from build123d import *

# Parameters (mm, degrees)
F1_DEPTH = 254
F2_R     = 2
F3_R     = 5


with BuildPart() as f1:
    # F0 (on Right) → F1 (new body)
    with BuildSketch(Plane.YZ):
        Polygon((-11.62, 7.9759603159), (-15.94, 12.2959603159), (-15.94, -0.5893383893), (-11.62, -0.5893383893), align=None)
        Polygon((-11.62, 11.0306616107), (-15.94, 15.3506616107), (-15.94, 12.2959603159), (-11.62, 7.9759603159), (-8.7938307864, 5.1497911023), (-7.266480139, 6.6771417497), align=None)
        Polygon((-8.5652987053, 11.0306616107), (-11.62, 11.0306616107), (-7.266480139, 6.6771417497), (-5.7391294917, 8.2044923971), align=None)
        Polygon((0, 15.3506616107), (-12.8852987053, 15.3506616107), (-8.5652987053, 11.0306616107), (0, 11.0306616107), align=None)
        Polygon((-12.8852987053, 15.3506616107), (-15.94, 15.3506616107), (-11.62, 11.0306616107), (-8.5652987053, 11.0306616107), align=None)
        Polygon((-15.94, -21.5946370946), (-11.62, -17.2746370946), (-11.62, -8.7093383893), (-15.94, -8.7093383893), align=None)
        Polygon((-3.625, -12.3343383893), (-3.625, -9.2796370946), (-11.62, -17.2746370946), (-15.94, -21.5946370946), (-15.94, -24.6493383893), (-12.8852987053, -24.6493383893), (-8.5652987053, -20.3293383893), (-0.5702987053, -12.3343383893), align=None)
        Polygon((0, -20.3293383893), (-8.5652987053, -20.3293383893), (-12.8852987053, -24.6493383893), (0, -24.6493383893), align=None)
        Polygon((14.9650698751, 9.3104327805), (8.6902987053, 3.0356616107), (11.745, 3.0356616107), (11.745, -0.0190396841), (18.0197711699, 6.2557314858), (19.74, 7.9759603159), (16.6852987053, 11.0306616107), align=None)
        Polygon((21.0052987053, 15.3506616107), (16.6852987053, 11.0306616107), (19.74, 7.9759603159), (24.06, 12.2959603159), (24.06, 15.3506616107), align=None)
        Polygon((24.06, 12.2959603159), (19.74, 7.9759603159), (19.74, -0.5893383893), (24.06, -0.5893383893), align=None)
        Polygon((8.12, 11.0306616107), (16.6852987053, 11.0306616107), (21.0052987053, 15.3506616107), (8.12, 15.3506616107), align=None)
        with BuildLine():
            Line((11.745, -9.2796370946), (11.745, -0.0190396841))
            Line((11.745, -0.0190396841), (7.4440143218, -4.3200253623))
            ThreePointArc((7.4440143218, -4.3200253623), (7.456001229, -4.4844879937), (7.46, -4.6493383893))
            ThreePointArc((7.46, -4.6493383893), (7.456001229, -4.8141887849), (7.4440143218, -4.9786514164))
            Line((7.4440143218, -4.9786514164), (11.745, -9.2796370946))
        make_face()
        with BuildLine():
            Line((3.7306869729, -8.0333527111), (-0.5702987053, -12.3343383893))
            Line((-0.5702987053, -12.3343383893), (8.6902987053, -12.3343383893))
            Line((8.6902987053, -12.3343383893), (4.3893130271, -8.0333527111))
            ThreePointArc((4.3893130271, -8.0333527111), (4.06, -8.0493383893), (3.7306869729, -8.0333527111))
        make_face()
        with BuildLine():
            Line((0.6759856782, -4.3200253623), (-3.625, -0.0190396841))
            Line((-3.625, -0.0190396841), (-3.625, -9.2796370946))
            Line((-3.625, -9.2796370946), (0.6759856782, -4.9786514164))
            ThreePointArc((0.6759856782, -4.9786514164), (0.66, -4.6493383893), (0.6759856782, -4.3200253623))
        make_face()
        with BuildLine():
            Line((8.6902987053, 3.0356616107), (-0.5702987053, 3.0356616107))
            Line((-0.5702987053, 3.0356616107), (3.7306869729, -1.2653240675))
            ThreePointArc((3.7306869729, -1.2653240675), (4.06, -1.2493383893), (4.3893130271, -1.2653240675))
            Line((4.3893130271, -1.2653240675), (8.6902987053, 3.0356616107))
        make_face()
        Polygon((-5.7391294917, 8.2044923971), (-7.266480139, 6.6771417497), (-3.625, 3.0356616107), (-0.5702987053, 3.0356616107), align=None)
        Polygon((-3.625, 3.0356616107), (-7.266480139, 6.6771417497), (-8.7938307864, 5.1497911023), (-3.625, -0.0190396841), align=None)
        Polygon((11.745, -12.3343383893), (8.6902987053, -12.3343383893), (16.6852987053, -20.3293383893), (21.0052987053, -24.6493383893), (24.06, -24.6493383893), align=None)
        Polygon((19.74, -17.2746370946), (11.745, -9.2796370946), (11.745, -12.3343383893), (24.06, -24.6493383893), (24.06, -21.5946370946), align=None)
        Polygon((19.74, -8.7093383893), (19.74, -17.2746370946), (24.06, -21.5946370946), (24.06, -8.7093383893), align=None)
        Polygon((21.0052987053, -24.6493383893), (16.6852987053, -20.3293383893), (8.12, -20.3293383893), (8.12, -24.6493383893), align=None)
        with BuildLine():
            Line((11.745, 3.0356616107), (8.6902987053, 3.0356616107))
            Line((8.6902987053, 3.0356616107), (4.3893130271, -1.2653240675))
            ThreePointArc((4.3893130271, -1.2653240675), (6.464163056, -2.2451753333), (7.4440143218, -4.3200253623))
            Line((7.4440143218, -4.3200253623), (11.745, -0.0190396841))
            Line((11.745, -0.0190396841), (11.745, 3.0356616107))
        make_face()
        with BuildLine():
            Line((1.655836944, -2.2451753333), (-3.625, 3.0356616107))
            Line((-3.625, 3.0356616107), (-3.625, -0.0190396841))
            Line((-3.625, -0.0190396841), (0.6759856782, -4.3200253623))
            ThreePointArc((0.6759856782, -4.3200253623), (0.9855894874, -3.1974430763), (1.655836944, -2.2451753333))
        make_face()
        with BuildLine():
            Line((0.6759856782, -4.9786514164), (-3.625, -9.2796370946))
            Line((-3.625, -9.2796370946), (-3.625, -12.3343383893))
            Line((-3.625, -12.3343383893), (-0.5702987053, -12.3343383893))
            Line((-0.5702987053, -12.3343383893), (3.7306869729, -8.0333527111))
            ThreePointArc((3.7306869729, -8.0333527111), (1.655836944, -7.0535014454), (0.6759856782, -4.9786514164))
        make_face()
        with BuildLine():
            Line((11.745, -12.3343383893), (6.464163056, -7.0535014454))
            ThreePointArc((6.464163056, -7.0535014454), (5.511895313, -7.7237489019), (4.3893130271, -8.0333527111))
            Line((4.3893130271, -8.0333527111), (8.6902987053, -12.3343383893))
            Line((8.6902987053, -12.3343383893), (11.745, -12.3343383893))
        make_face()
        with BuildLine():
            ThreePointArc((7.4440143218, -4.9786514164), (7.1344105126, -6.1012337024), (6.464163056, -7.0535014454))
            Line((6.464163056, -7.0535014454), (11.745, -12.3343383893))
            Line((11.745, -12.3343383893), (11.745, -9.2796370946))
            Line((11.745, -9.2796370946), (7.4440143218, -4.9786514164))
        make_face()
        with BuildLine():
            Line((-0.5702987053, 3.0356616107), (-3.625, 3.0356616107))
            Line((-3.625, 3.0356616107), (1.655836944, -2.2451753333))
            ThreePointArc((1.655836944, -2.2451753333), (2.608104687, -1.5749278767), (3.7306869729, -1.2653240675))
            Line((3.7306869729, -1.2653240675), (-0.5702987053, 3.0356616107))
        make_face()
    extrude(amount=F1_DEPTH)

    # F2
    f2_edges = [f1.edges().sort_by_distance(p)[0] for p in [
        (127, 0, 11.030662),
        (127, -11.62, -0.589338),
        (127, -15.94, -0.589338),
        (127, 0, 15.350662),
        (127, 8.12, 11.030662),
        (127, 19.74, -0.589338),
        (127, 24.06, -0.589338),
        (127, 8.12, -24.649338),
        (127, 8.12, 15.350662),
        (127, -15.94, -8.709338),
        (127, -11.62, -8.709338),
        (127, 0, -24.649338),
        (127, 0, -20.329338),
        (127, 8.12, -20.329338),
        (127, 19.74, -8.709338),
        (127, 24.06, -8.709338),
    ]]
    fillet(f2_edges, radius=F2_R)

    # F3
    f3_edges = [f1.edges().sort_by_distance(p)[0] for p in [
        (127, -15.94, 15.350662),
        (127, 24.06, 15.350662),
        (127, 24.06, -24.649338),
        (127, -15.94, -24.649338),
    ]]
    fillet(f3_edges, radius=F3_R)


solid = f1.part
Geometry: final body of the model. Coordinates: model frame, mm. Round coordinates to 2 decimals unless told otherwise and drop trailing zeros. Write item = value, one per line.
Item 1: Material intervals for line 1 along Z through (x, y) = (219, -5.5); line 2 along Z through (x, y) = (122.5, 10); line 3 along Z through (x, y) = (167, 13.5), sorted ascending. Write a range as [from, to].
Findings:
line_1 = [-24.65, -20.33], [-17.26, -11.15], [1.86, 7.97], [11.03, 15.35]
line_2 = [-24.65, -20.33], [-13.64, 4.35], [11.03, 15.35]
line_3 = [-24.65, -20.33], [-17.14, -11.03], [1.74, 7.85], [11.03, 15.35]
Item 2: Pull-direction query (Z, two-part tool) for faces 1 (the face through (125, 19.74, -14)), 2 (the face through (125, 15, 15.351)), 3 (the face through (0, -1, -4)); classes: pulls with the +Z half, pulls with the -Z half, needs draft (parallel to the pull), parting line crosses it, or undercut.
Findings:
face_1 = undercut
face_2 = pulls with the +Z half
face_3 = needs draft
Item 3: Pin query (flat end, axial travel): P1, Ø4.5, axis at x = 184.5, y = 5.5, coming from the +Z side; P2, Ø3, axis at x = 73, z = -1.5, coming from the -Y side; P3, Ø10, axis at x = 78.5, z = -5.5, coming from the +Y side. Return the tip coordinate at first contact, or that it passes through.
Findings:
P1 = 3.04
P2 = -15.36
P3 = 24.05
